Print and shaded views of the part. All mm, measured from the part's lowest x, y and z. A direction names the side the tool comes from. Coordinates: 2 decimals unless noted, no trailing zeros. Loops run counter-clockwise (first coordinate to the right, second up) from the corner with the lowest first, then second, coordinate; pieces in that order, holes last.
1) Saw through at A-A, the plane y = 24. Give the number of separate pieces and of enclosed holes in the cut face, and give its area (3 significant figures).
2) Which spindle directions (+Z, -Z, +X, -X, +Y, -Y) get a long thin tool onto all of the face, cutting with end or side? Do the marked faces 1 and 2. Say none if no direction does.
3) Saw through at B-B, the plane x = 22.5. Write the cut outline in (y, z).
4) Wall check: line 1 along X through (y, z) = (43, 6.5). Give the ranges that are in metal, low to high.
5) Two-plate mould, pull along Y, no slides. Class the marked faces 3, 4 and 5: +Y half, -Y half, draft (parallel to the pull), parting line (faces both ways), or undercut.
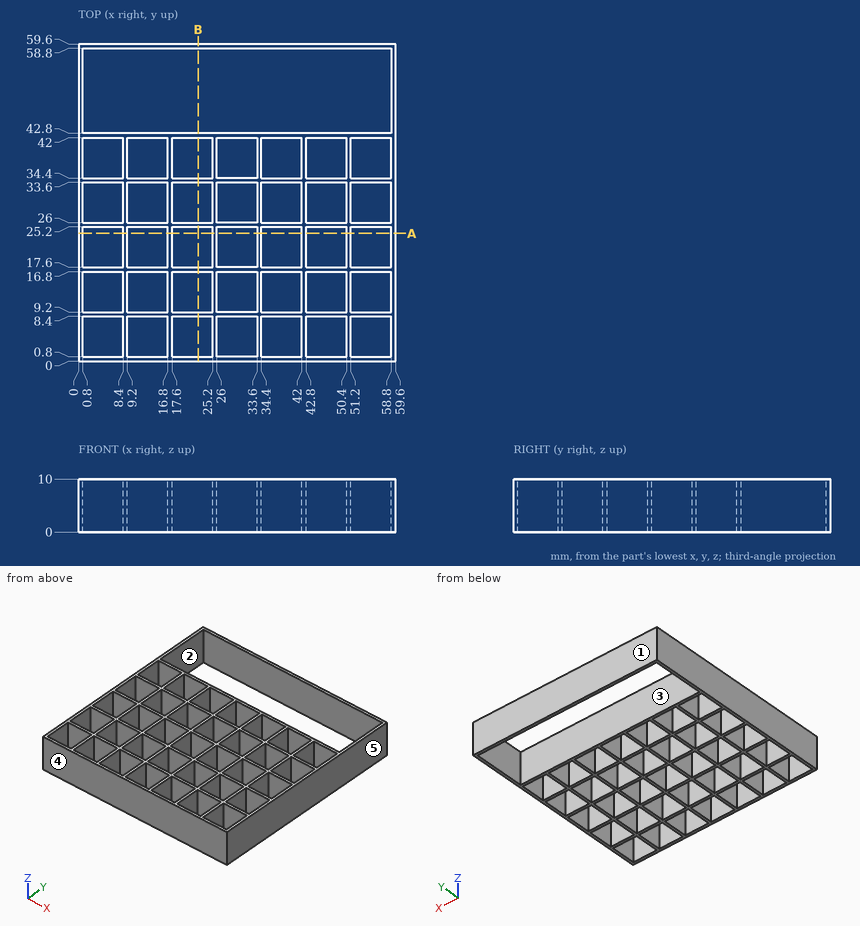
Data:
1. separate pieces: 8
1. enclosed holes: 0
1. area: 64.0 mm2
2. face 1: +Z, -Z, +X, -X, +Y
2. face 2: +Z, -Z
3. outline: (0, 0) - (0.8, 0) - (0.8, 10) - (0, 10) - close; (8.4, 0) - (9.2, 0) - (9.2, 10) - (8.4, 10) - close; (16.8, 0) - (17.6, 0) - (17.6, 10) - (16.8, 10) - close; (25.2, 0) - (26, 0) - (26, 10) - (25.2, 10) - close; (33.6, 0) - (34.4, 0) - (34.4, 10) - (33.6, 10) - close; (42, 0) - (42.8, 0) - (42.8, 10) - (42, 10) - close; (58.8, 0) - (59.6, 0) - (59.6, 10) - (58.8, 10) - close
4. line 1: x = 0 to 0.8, 58.8 to 59.6
5. face 3: undercut
5. face 4: -Y half
5. face 5: draft
